```python
from build123d import *

# Parameters (mm, degrees)
BOSS_EXTRUDE1_DEPTH  = 3
M5_CLEARANCE_HOLE1_D = 5.5
M5_CLEARANCE_HOLE2_D = 5.5
M5_CLEARANCE_HOLE3_D = 5.5


with BuildPart() as part:
    # Sketch1 → Boss-Extrude1 (new body)
    with BuildSketch(Plane.XY):
        with BuildLine():
            Line((-51.88, -9.5), (0, -9.5))
            ThreePointArc((0, -9.5), (9.5, 0), (0, 9.5))
            Line((0, 9.5), (-51.88, 9.5))
            Line((-51.88, 9.5), (-51.88, -9.5))
        make_face()
    extrude(amount=BOSS_EXTRUDE1_DEPTH)

    # M5 Clearance Hole1 (through all)
    with Locations(Plane.XY.offset(3)):
        with Locations((-43.44, 0)):
            Hole(M5_CLEARANCE_HOLE1_D / 2)

    # M5 Clearance Hole2 (through all)
    with Locations(Plane.XY.offset(3)):
        with Locations((-23.44, 0)):
            Hole(M5_CLEARANCE_HOLE2_D / 2)

    # M5 Clearance Hole3 (through all)
    with Locations(Plane.XY.offset(3)):
        with Locations((0, 0)):
            Hole(M5_CLEARANCE_HOLE3_D / 2)


solid = part.part
```
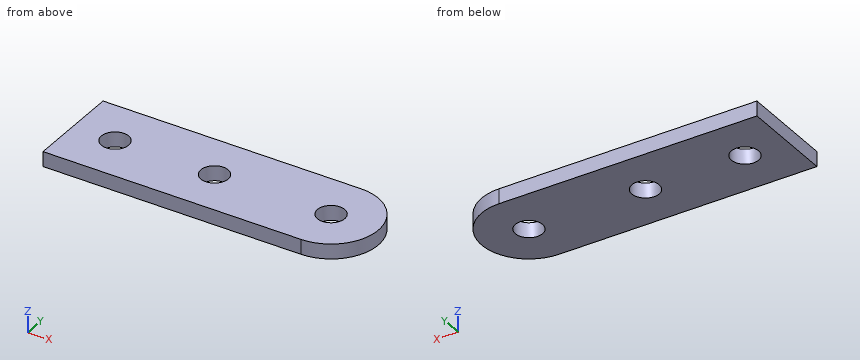
Input: part model. Units: mm. Frame: model coordinates. Coordinates: 2 decimals unless noted, no trailing zeros. Loops run counter-clockwise (first coordinate to the right, second up) from the corner with the lowest first, then second, coordinate; pieces in that order, holes last. Notation, with made-up numbers: M 4,9 L 23,9 A18 ccw 23,32 Z; hole C 5,69.5 d2. An arc over 180 degrees is marked long. Use a Markdown table: item, result. Add a question column.
1) Section A-A, the plane z = 0.6. Return the cut outline in (x, y), plus the area to 3 significant figures.
2) Section D-D, the plane y = 6. Return the cut outline in (x, z), plus the area to 3 significant figures.
3) Section C-C, the plane x = -23.44. Return the cut outline in (y, z).
4) Section B-B, the plane y = 0. Return the cut outline in (x, z), plus the area to 3 significant figures.
5) Line query: L1, parallel to Y at x = -23.44, z = 1.8; L2, parallel to X at y = 2.25, z = 0.4; L3, parallel to Y at x = 2, z = 2.75. Output: solid intervals per line, ascending. Write a range as from..to.
Answer below:
| question | item | result |
|---|---|---|
| 1 | outline | M -51.88,-9.5 L 0,-9.5 A9.5 ccw 0,9.5 L -51.88,9.5 Z; hole C -43.44,0 d5.5; hole C -23.44,0 d5.5; hole C 0,0 d5.5 |
| 1 | area | 1,060 mm2 |
| 2 | outline | M -51.88,0 L 7.37,0 L 7.37,3 L -51.88,3 Z |
| 2 | area | 178 mm2 |
| 3 | outline | M -9.5,0 L -2.75,0 L -2.75,3 L -9.5,3 Z; M 2.75,0 L 9.5,0 L 9.5,3 L 2.75,3 Z |
| 4 | outline | M -51.88,0 L -46.19,0 L -46.19,3 L -51.88,3 Z; M -40.69,0 L -26.19,0 L -26.19,3 L -40.69,3 Z; M -20.69,0 L -2.75,0 L -2.75,3 L -20.69,3 Z; M 2.75,0 L 9.5,0 L 9.5,3 L 2.75,3 Z |
| 4 | area | 135 mm2 |
| 5 | L1 | -9.5..-2.75, 2.75..9.5 |
| 5 | L2 | -51.88..-45.02, -41.86..-25.02, -21.86..-1.58, 1.58..9.23 |
| 5 | L3 | -9.29..-1.89, 1.89..9.29 |
